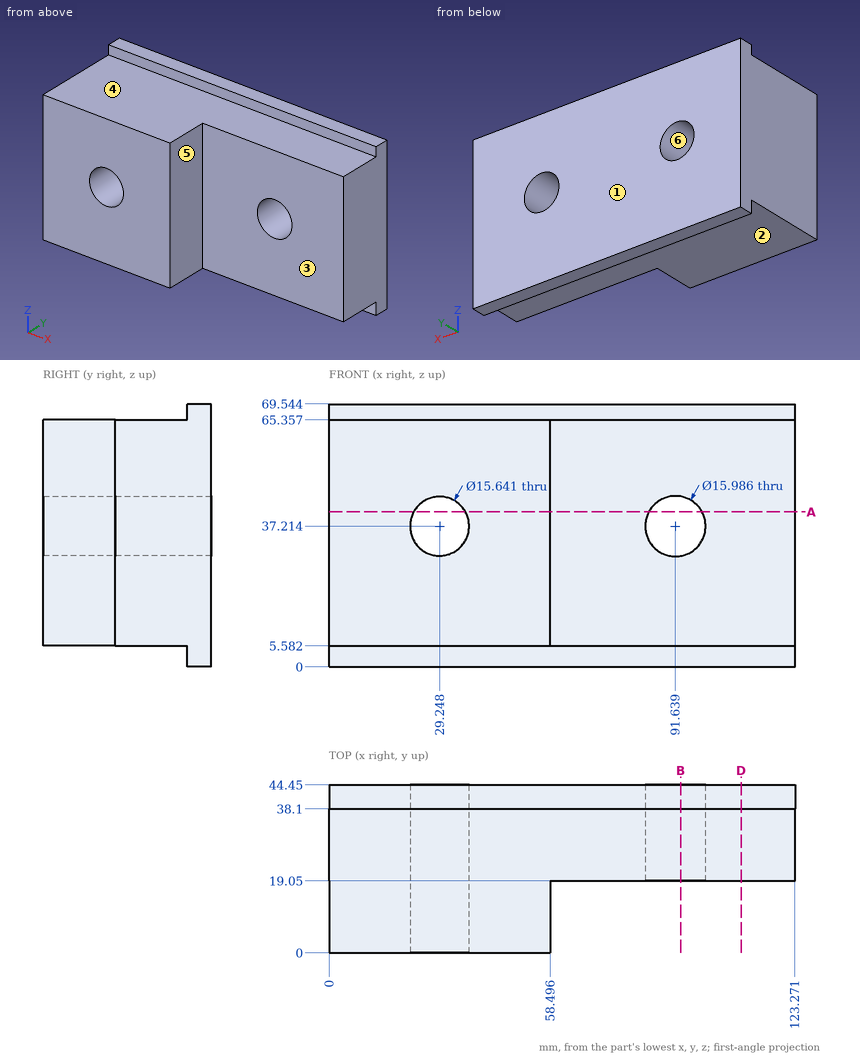
Check sheet for the drawn part. Datum: minimum x, y, z corner. Units: mm. A direction names the side the tool comes from. Coordinates: 2 decimals unless noted, no trailing zeros. Write each loop counter-clockwise with the first axis right and the second up, starting at its lowest first coordinate (ties: lowest second). Pieces come first, ordered by that corner, then holes. Notation, with made-up numbers: M 16,84.5 L 38,84.5 A17 cw 38,108.5 Z; hole C 38,34.25 d8. An arc over 180 degrees is marked long. One line per item, written item: value.
Item 1: Section check B-B, the plane x = 93. Record the boundary of the cut face in (y, z).
Check sheet entries:
outline: M 19.05,5.58 L 38.1,5.58 L 38.1,0 L 44.45,0 L 44.45,29.34 L 19.05,29.34 Z; M 19.05,45.09 L 44.45,45.09 L 44.45,69.54 L 38.1,69.54 L 38.1,65.36 L 19.05,65.36 Z
Item 2: Gauge pin test, flat ends, axial feed: pin 1 Ø3 at (x, y) = (79, 35) entering from -Z; pin 2 Ø5.5 at (y, z) = (8.5, 40) entering from +X; pin 3 Ø1.7 at (x, z) = (64, 3) entering from -Y. Record the tip position at first contact, or that the pin passes through.
Check sheet entries:
pin 1: stops at z = 5.58
pin 2: stops at x = 58.5
pin 3: stops at y = 38.1
Item 3: Access from +Z, -Z, +X, -X, +Y, -Y to the whole of each face (thin tool, end or side, straight path). Record for the marked faces 1, 2 and 3.
Check sheet entries:
face 1: +Z, -Z, +X, -X, +Y
face 2: -Z, +X, -X, -Y
face 3: +Z, -Z, +X, -Y
Item 4: Scan lines: line 1 along X through (y, z) = (30, 34); line 2 along X through (y, z) = (10, 56) (1 decimal); line 3 along Z through (x, y) = (58, 33). Record each from-to range of solid material in increasing order.
Check sheet entries:
line 1: x = 0 to 22.12, 36.38 to 84.32, 98.96 to 123.27
line 2: x = 0 to 58.5
line 3: z = 5.58 to 65.36
Item 5: Section check D-D, the plane x = 109. Record the boundary of the cut face in (y, z).
Check sheet entries:
outline: M 19.05,5.58 L 38.1,5.58 L 38.1,0 L 44.45,0 L 44.45,69.54 L 38.1,69.54 L 38.1,65.36 L 19.05,65.36 Z
Item 6: Section check A-A, the plane z = 41. State how many separate pieces and enclosed holes the cut face has, plus the area to 3 significant figures.
Check sheet entries:
separate pieces: 3
enclosed holes: 0
area: 3,280 mm^2
Item 7: Mould release check, pull along Z, two halves, no side actions. Record for the marked faces 4, 5 and 6: pulls with the +Z half, pulls with the -Z half, needs draft (parallel to the pull), parting line crosses it, or undercut.
Check sheet entries:
face 4: pulls with the +Z half
face 5: needs draft
face 6: undercut
